Could you check a few things on this model? Use its own coordinates, in mm. A direction names the side the tool comes from. Give positions to 0.01 mm unless a question says otherwise; leave off trailing zeros. Use one line per item in the form item = value. Start each with the question number.
from build123d import *

# Parameters (mm, degrees)
F1_DEPTH = 240
F2_R     = 1.5
F3_R     = 0.5


with BuildPart() as f1:
    # F0 (on Top) → F1 (new body)
    with BuildSketch(Plane.XY):
        Polygon((-2.6, 8.5), (-2.6, 10), (-10, 10), (-10, 2.6), (-8.5, 2.6), (-8.5, 6), (-8.5, 7.4393398282), (-8.5, 8.5), (-7.4393398282, 8.5), (-6, 8.5), align=None)
        Polygon((-8.5, 7.4393398282), (-8.5, 6), (-7.0606601718, 6), align=None)
        Polygon((-6, 7.0606601718), (-6, 8.5), (-7.4393398282, 8.5), align=None)
        Polygon((-6, 7.0606601718), (-7.4393398282, 8.5), (-8.5, 8.5), (-8.5, 7.4393398282), (-7.0606601718, 6), (-3.65, 2.5893398282), (-3.65, 3.65), (-2.5893398282, 3.65), align=None)
        Polygon((10, 2.6), (10, 10), (2.6, 10), (2.6, 8.5), (6, 8.5), (7.4393398282, 8.5), (8.5, 8.5), (8.5, 7.4393398282), (8.5, 6), (8.5, 2.6), align=None)
        Polygon((7.4393398282, 8.5), (6, 8.5), (6, 7.0606601718), align=None)
        Polygon((8.5, 8.5), (7.4393398282, 8.5), (6, 7.0606601718), (2.5893398282, 3.65), (3.65, 3.65), (3.65, 2.5893398282), (7.0606601718, 6), (8.5, 7.4393398282), align=None)
        Polygon((7.0606601718, 6), (8.5, 6), (8.5, 7.4393398282), align=None)
        Polygon((6, -7.0606601718), (6, -8.5), (7.4393398282, -8.5), align=None)
        Polygon((8.5, -8.5), (8.5, -7.4393398282), (7.0606601718, -6), (3.65, -2.5893398282), (3.65, -3.65), (2.5893398282, -3.65), (6, -7.0606601718), (7.4393398282, -8.5), align=None)
        Polygon((8.5, -7.4393398282), (8.5, -6), (7.0606601718, -6), align=None)
        Polygon((10, -10), (10, -2.6), (8.5, -2.6), (8.5, -6), (8.5, -7.4393398282), (8.5, -8.5), (7.4393398282, -8.5), (6, -8.5), (2.6, -8.5), (2.6, -10), align=None)
        Polygon((-8.5, -2.6), (-10, -2.6), (-10, -10), (-2.6, -10), (-2.6, -8.5), (-6, -8.5), (-7.4393398282, -8.5), (-8.5, -8.5), (-8.5, -7.4393398282), (-8.5, -6), align=None)
        Polygon((-7.4393398282, -8.5), (-6, -8.5), (-6, -7.0606601718), align=None)
        Polygon((-7.0606601718, -6), (-8.5, -6), (-8.5, -7.4393398282), align=None)
        Polygon((-7.0606601718, -6), (-8.5, -7.4393398282), (-8.5, -8.5), (-7.4393398282, -8.5), (-6, -7.0606601718), (-2.5893398282, -3.65), (-3.65, -3.65), (-3.65, -2.5893398282), align=None)
        with BuildLine():
            Line((-2.4829614997, -1.4223013279), (-3.65, -2.5893398282))
            Line((-3.65, -2.5893398282), (-3.65, -3.65))
            Line((-3.65, -3.65), (-2.5893398282, -3.65))
            Line((-2.5893398282, -3.65), (-1.4223013279, -2.4829614997))
            ThreePointArc((-1.4223013279, -2.4829614997), (-2.1920310217, -2.1920310217), (-2.4829614997, -1.4223013279))
        make_face()
        with BuildLine():
            Line((-2.5893398282, -3.65), (2.5893398282, -3.65))
            Line((2.5893398282, -3.65), (1.4223013279, -2.4829614997))
            ThreePointArc((1.4223013279, -2.4829614997), (0.9671620585, -2.3404488298), (0.6297938115, -2.0033371546))
            ThreePointArc((0.6297938115, -2.0033371546), (0, -2.1), (-0.6297938115, -2.0033371546))
            ThreePointArc((-0.6297938115, -2.0033371546), (-0.9671620585, -2.3404488298), (-1.4223013279, -2.4829614997))
            Line((-1.4223013279, -2.4829614997), (-2.5893398282, -3.65))
        make_face()
        with BuildLine():
            Line((3.65, -3.65), (3.65, -2.5893398282))
            Line((3.65, -2.5893398282), (2.4829614997, -1.4223013279))
            ThreePointArc((2.4829614997, -1.4223013279), (2.4844334349, -1.4535974088), (2.4849242405, -1.4849242405))
            ThreePointArc((2.4849242405, -1.4849242405), (2.1695325546, -2.2138353848), (1.4223013279, -2.4829614997))
            Line((1.4223013279, -2.4829614997), (2.5893398282, -3.65))
            Line((2.5893398282, -3.65), (3.65, -3.65))
        make_face()
        with BuildLine():
            Line((3.65, -2.5893398282), (3.65, 2.5893398282))
            Line((3.65, 2.5893398282), (2.4829614997, 1.4223013279))
            ThreePointArc((2.4829614997, 1.4223013279), (2.3404488298, 0.9671620585), (2.0033371546, 0.6297938115))
            ThreePointArc((2.0033371546, 0.6297938115), (2.075693622, 0.3185843494), (2.1, 0))
            ThreePointArc((2.1, 0), (2.075693622, -0.3185843494), (2.0033371546, -0.6297938115))
            ThreePointArc((2.0033371546, -0.6297938115), (2.3404488298, -0.9671620585), (2.4829614997, -1.4223013279))
            Line((2.4829614997, -1.4223013279), (3.65, -2.5893398282))
        make_face()
        with BuildLine():
            Line((3.65, 3.65), (2.5893398282, 3.65))
            Line((2.5893398282, 3.65), (1.4223013279, 2.4829614997))
            ThreePointArc((1.4223013279, 2.4829614997), (2.1695325546, 2.2138353848), (2.4849242405, 1.4849242405))
            ThreePointArc((2.4849242405, 1.4849242405), (2.4844334349, 1.4535974088), (2.4829614997, 1.4223013279))
            Line((2.4829614997, 1.4223013279), (3.65, 2.5893398282))
            Line((3.65, 2.5893398282), (3.65, 3.65))
        make_face()
        with BuildLine():
            Line((1.4223013279, 2.4829614997), (2.5893398282, 3.65))
            Line((2.5893398282, 3.65), (-2.5893398282, 3.65))
            Line((-2.5893398282, 3.65), (-1.4223013279, 2.4829614997))
            ThreePointArc((-1.4223013279, 2.4829614997), (-0.9671620585, 2.3404488298), (-0.6297938115, 2.0033371546))
            ThreePointArc((-0.6297938115, 2.0033371546), (0, 2.1), (0.6297938115, 2.0033371546))
            ThreePointArc((0.6297938115, 2.0033371546), (0.9671620585, 2.3404488298), (1.4223013279, 2.4829614997))
        make_face()
        with BuildLine():
            Line((-1.4223013279, 2.4829614997), (-2.5893398282, 3.65))
            Line((-2.5893398282, 3.65), (-3.65, 3.65))
            Line((-3.65, 3.65), (-3.65, 2.5893398282))
            Line((-3.65, 2.5893398282), (-2.4829614997, 1.4223013279))
            ThreePointArc((-2.4829614997, 1.4223013279), (-2.1920310217, 2.1920310217), (-1.4223013279, 2.4829614997))
        make_face()
        with BuildLine():
            Line((-2.4829614997, 1.4223013279), (-3.65, 2.5893398282))
            Line((-3.65, 2.5893398282), (-3.65, -2.5893398282))
            Line((-3.65, -2.5893398282), (-2.4829614997, -1.4223013279))
            ThreePointArc((-2.4829614997, -1.4223013279), (-2.3404488298, -0.9671620585), (-2.0033371546, -0.6297938115))
            ThreePointArc((-2.0033371546, -0.6297938115), (-2.1, 0), (-2.0033371546, 0.6297938115))
            ThreePointArc((-2.0033371546, 0.6297938115), (-2.3404488298, 0.9671620585), (-2.4829614997, 1.4223013279))
        make_face()
    extrude(amount=-F1_DEPTH)

    # F2
    f2_edges = [f1.edges().sort_by_distance(p)[0] for p in [
        (-10, -10, -120),
        (-10, 10, -120),
        (10, -10, -120),
        (10, 10, -120),
    ]]
    fillet(f2_edges, radius=F2_R)

    # F3
    f3_edges = [f1.edges().sort_by_distance(p)[0] for p in [
        (-6, -8.5, -120),
        (-8.5, -6, -120),
        (-8.5, 6, -120),
        (-6, 8.5, -120),
        (6, -8.5, -120),
        (8.5, -6, -120),
        (8.5, 6, -120),
        (6, 8.5, -120),
        (-2.6, 10, -120),
        (-2.6, 8.5, -120),
        (2.6, 10, -120),
        (-8.5, 2.6, -120),
        (-8.5, -2.6, -120),
        (-10, -2.6, -120),
        (-2.6, -8.5, -120),
        (-2.6, -10, -120),
        (2.6, -8.5, -120),
        (8.5, -2.6, -120),
        (10, -2.6, -120),
        (10, 2.6, -120),
        (8.5, 2.6, -120),
        (2.6, 8.5, -120),
        (-10, 2.6, -120),
        (2.6, -10, -120),
    ]]
    fillet(f3_edges, radius=F3_R)


solid = f1.part
(1) We'd pull the mould along Y, two halves only. Please class faces 4 (the flat face through (-10, 6, -118)), 5 (the flat face through (0, 3.65, -118)), 6 (the flat face through (-3.65, 0, -118)): pulls with the +Y half, pulls with the -Y half, needs draft (parallel to the pull), parting line crosses it, or undercut.
(2) I'm going to push flat-ended pins straight in: pin 1 Ø1.6 at (y, z) = (-1, -162) entering from +X; pin 2 Ø1.6 at (y, z) = (-0.5, -142.5) entering from -X; pin 3 Ø0.6 at (x, z) = (-9, -107.5) entering from -Y. Where does each tip first touch, or does it pass through?
(3) Please list where these lines run through material, in increasing order: probe 1 along X at (y, z) = (8, -13.5); probe 2 along X at (y, z) = (-4.75, -85.5).
(4) Which directions (+Z, -Z, +X, -X, +Y, -Y) give clear straight access to the entire face, cutting with the end or side of a thin tool? Please do faces 1 (the flat face through (10, 6, -118)), 2 (the flat face through (0, -3.65, -118)), 3 (the flat face through (3.65, 0, -118)).
Calculated:
q1.face_4 = needs draft
q1.face_5 = pulls with the +Y half
q1.face_6 = undercut
q2.pin_1 = 3.65
q2.pin_2 = -3.65
q2.pin_3 = -9.99
q3.probe_1 = -10 to -6, 6 to 10
q3.probe_2 = -10 to -8.5, -5.81 to -3.69, 3.69 to 5.81, 8.5 to 10
q4.face_1 = +Z, -Z, +X, +Y, -Y
q4.face_2 = +Z, -Z, -Y
q4.face_3 = +Z, -Z, +X
